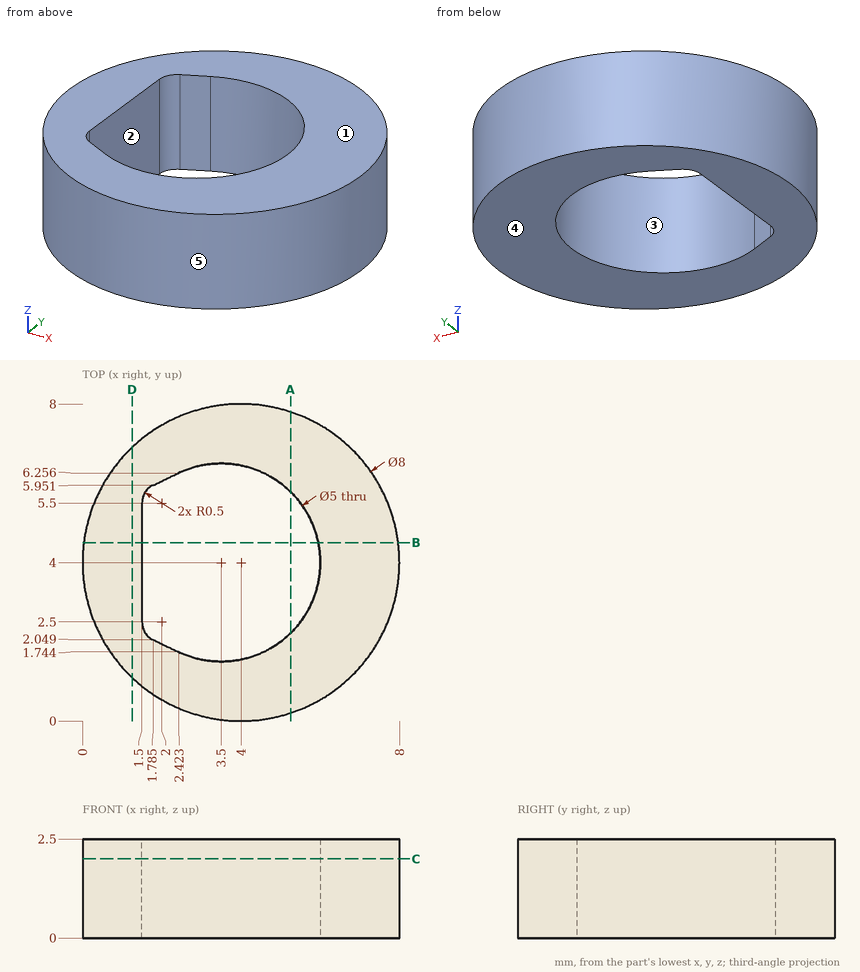
The figure shows three views and two pictorial views of one solid part (mm, origin at its lowest corner). Answer the questions. A direction names the side the tool comes from. Round coordinates to 2 decimals unless told otherwise and drop trailing zeros. Write each loop counter-clockwise with the first axis right and the second up, starting at its lowest first coordinate (ties: lowest second). Pieces come first, ordered by that corner, then holes. Notation, with made-up numbers: (-35, 3.25) - (10, 3.25) arc R20 ccw to (10, 32.25) - close; hole circle Ø10 at (33.5, 56.5). An arc over 180 degrees is marked (long way). Answer in a Markdown table with one row per item. Add a question column.
1. A cutting plane is placed at B-B, the plane y = 4.5. Determine the outline of the cut face in (x, z).
2. For the marked faces 1 and 2, determine the directions among +Z, -Z, +X, -X, +Y, -Y from which every point of the face is accessible in a straight line to the end or side of a thin tool.
3. The mould has two halves that part along Y. Classify the marked faces 3, 4 and 5: +Y half, -Y half, draft (parallel to the pull), parting line (faces both ways), or undercut.
4. A cutting plane is placed at C-C, the plane z = 2. Determine the outline of the cut face in (x, y) (1 decimal).
5. A cutting plane is placed at D-D, the plane x = 1.25. Determine the outline of the cut face in (y, z) (1 decimal).
6. Given pin 1 (1.5 mm diameter, centred on y = 3, z = 0.5, fed in from -X); pin 2 (1 mm diameter, centred on x = 7, z = 1, fed in from -Y); pin 3 (1.5 mm diameter, centred on x = 6, z = 0.5, fed in from -Y), each flat-ended and moving along its own axis, determine where each tip first touches the part or whether it passes through.
7. Find the intervals of material crossed by line 1 along Y through (x, z) = (3.5, 1.75); line 2 along X through (y, z) = (6.25, 1.3) (1 decimal); line 3 along X through (y, z) = (5.75, 1.5) (1 decimal), in increasing order. Write a range as from..to.
8. A cutting plane is placed at A-A, the plane x = 5.25. Determine the outline of the cut face in (y, z) (1 decimal), and give its area (3 significant figures).
Worked out:
| question | item | result |
|---|---|---|
| 1 | outline | (0.03, 0) - (1.5, 0) - (1.5, 2.5) - (0.03, 2.5) - close; (5.95, 0) - (7.97, 0) - (7.97, 2.5) - (5.95, 2.5) - close |
| 2 | face 1 | +Z, +X, -X, +Y, -Y |
| 2 | face 2 | +Z, -Z |
| 3 | face 3 | undercut |
| 3 | face 4 | draft |
| 3 | face 5 | parting line |
| 4 | outline | circle Ø8 at (4, 4); hole (1.5, 2.5) arc R0.5 ccw to (1.8, 2) - (2.4, 1.7) arc R2.5 ccw (long way) to (2.4, 6.3) - (1.8, 6) arc R0.5 ccw to (1.5, 5.5) - close |
| 5 | outline | (1.1, 0) - (6.9, 0) - (6.9, 2.5) - (1.1, 2.5) - close |
| 6 | pin 1 | x = 0.01 |
| 6 | pin 2 | y = 0.88 |
| 6 | pin 3 | y = 0.2 |
| 7 | line 1 | 0.03..1.5, 6.5..7.97 |
| 7 | line 2 | 0.7..2.4, 4.6..7.3 |
| 7 | line 3 | 0.4..1.6, 5.3..7.6 |
| 8 | outline | (0.2, 0) - (2.2, 0) - (2.2, 2.5) - (0.2, 2.5) - close; (5.8, 0) - (7.8, 0) - (7.8, 2.5) - (5.8, 2.5) - close |
| 8 | area | 10.1 mm^2 |
